The model under review builds one solid part; all positions refer to its coordinate system, in mm. Round coordinates to 2 decimals unless told otherwise and drop trailing zeros. Write each loop counter-clockwise with the first axis right and the second up, starting at its lowest first coordinate (ties: lowest second). Pieces come first, ordered by that corner, then holes. Notation, with made-up numbers: (74, 84) - (106, 84) arc R14 ccw to (106, 99) - close; hole circle Ø9 at (-37.5, -12.5). An arc over 180 degrees is marked (long way). Return JSON: item names as keys, results as strings.
from build123d import *

# Parameters (mm, degrees)
SKETCH1_R           = 3.175
SKETCH1_R_2         = 2.25
BOSS_EXTRUDE1_DEPTH = 45.72
SKETCH2_W           = 3.810610938
SKETCH2_H           = 3.347268665
CUT_EXTRUDE1_DEPTH  = 48.514
SKETCH3_R           = 1.5
CUT_EXTRUDE2_DEPTH  = 2.54


with BuildPart() as part:
    # Sketch1 → Boss-Extrude1 (new body)
    with BuildSketch(Plane.XY):
        Circle(SKETCH1_R)
        Circle(SKETCH1_R_2, mode=Mode.SUBTRACT)
    extrude(amount=BOSS_EXTRUDE1_DEPTH)

    # Sketch2 → Cut-Extrude1 (cut)
    with BuildSketch(Plane.XY.offset(45.72)):
        with Locations((0.085656613, 4.275461199)):
            Rectangle(SKETCH2_W, SKETCH2_H)
    extrude(amount=-CUT_EXTRUDE1_DEPTH, mode=Mode.SUBTRACT)

    # Sketch3 → Cut-Extrude2 (cut)
    with BuildSketch(Plane(origin=(0, 2.601826866, 0), x_dir=(1, 0, 0), z_dir=(0, 1, 0))):
        with Locations(Location((0, -3.81, 0), (0, 0, 270))):
            Circle(SKETCH3_R)
    extrude(amount=-CUT_EXTRUDE2_DEPTH, mode=Mode.SUBTRACT)


solid = part.part
(1) Mouldability with a two-part tool opening along X and no side actions: class faces 1 (the cylindrical face through (-0.112, -3.173, 22.54)), 2 (the cylindrical face through (-1.33, 2.25, 4.5)), 3 (the flat face through (1.4, -2.2, 0)) as released by +X, released by -X, zero draft, split by the parting line, or undercut.
Filled in:
{"face 1": "split by the parting line", "face 2": "undercut", "face 3": "zero draft"}
(2) Wall thickness on line 1 (Z direction, x = 0, y = 2.4); line 2 (X direction, y = -0.7, z = 18); line 3 (Y direction, x = -1.75, z = 15): over which ranges is each line inside the solid? List them lowest first.
Filled in:
{"line 1": "z = 0 to 2.31, 5.31 to 45.72", "line 2": "x = -3.1 to -2.14, 2.14 to 3.1", "line 3": "y = -2.65 to -1.41, 1.41 to 2.6"}
(3) Clearance check with flat-ended pins moving along their axes: pin 1 Ø1 at (x, z) = (-1.5, 18.5) entering from -Y; pin 2 Ø1 at (x, z) = (2, 27) entering from -Y. State where each tip first meets the part, or that it passes through.
Filled in:
{"pin 1": "stops at y = -3.01", "pin 2": "stops at y = -2.8"}
(4) Add section A-A (x = 0). Write out the cut boundary in (y, z) (3 decimals).
Filled in:
{"outline": "(-3.175, 0) - (-2.25, 0) - (-2.25, 45.72) - (-3.175, 45.72) - close; (2.25, 0) - (2.602, 0) - (2.602, 2.31) - (2.25, 2.31) - close; (2.25, 5.31) - (2.602, 5.31) - (2.602, 45.72) - (2.25, 45.72) - close"}
(5) Add section B-B (y = 0). Write out the cut boundary in (x, z) (3 decimals).
Filled in:
{"outline": "(-3.175, 0) - (-2.25, 0) - (-2.25, 45.72) - (-3.175, 45.72) - close; (2.25, 0) - (3.175, 0) - (3.175, 45.72) - (2.25, 45.72) - close"}
(6) Add section D-D (z = 3.81). Write out the cut boundary in (x, y) (3 decimals), plus the area to 3 significant figures.
Filled in:
{"outline": "(-1.82, 2.602) arc R3.175 ccw (long way) to (1.82, 2.602) - (1.5, 2.602) - (1.5, 1.677) arc R2.25 cw (long way) to (-1.5, 1.677) - (-1.5, 2.602) - close", "area": "12.8 mm2"}
(7) Add section C-C (z = 16.5). Write out the cut boundary in (x, y) (3 decimals).
Filled in:
{"outline": "(-1.82, 2.602) arc R3.175 ccw (long way) to (1.82, 2.602) - close; hole circle Ø4.5 at (0, 0)"}
